Geometry: final body of the model. Coordinates: model frame, mm. A direction names the side the tool comes from. Give positions to 0.01 mm unless a question says otherwise; leave off trailing zeros. Loops run counter-clockwise (first coordinate to the right, second up) from the corner with the lowest first, then second, coordinate; pieces in that order, holes last.
1. Section A-A, the plane x = 135. Output: boundary loops of the cut face in (y, z), then the cut area to 3 significant figures.
2. Material intervals for line 1 along X through (y, z) = (3.25, -9); line 2 along Y through (x, z) = (135, -76.8); line 3 along X through (y, z) = (5, -88.25), sorted ascending.
3. Access query for faces 5 (the face through (15, 5, -15)), 6 (the face through (74, 10, -46)), 7 (the face through (131, 5, -82)), 8 (the face through (74, 5, -90)), 9 (the face through (137.86, 4.1, -77.41)). Directions: +Z, -Z, +X, -X, +Y, -Y. A direction counts if a zero-diameter tool reaches every point of the face in a straight line with its end or side. Return the directions, or none.
4. First-contact query: P1, Ø3, axis at x = 15, y = 5, coming from the -Z side; P2, Ø3.5, axis at x = 135, y = 5, coming from the +Z side. Flat tips, straight axial feed; report the tip coordinate or a pass-through.
5. Draft query along Z for faces 1 (the face through (74, 5, 0)), 2 (the face through (131, 5, -8)), 3 (the face through (135, 5, -75)), 4 (the face through (0, 5, -44)). Return one class per face: +Z half, -Z half, draft (parallel to the pull), parting line (faces both ways), or undercut.
from build123d import *

# Parameters (mm, degrees)
SKETCH1_W           = 150
SKETCH1_H           = 90
SKETCH1_W_2         = 8
SKETCH1_H_2         = 4
BOSS_EXTRUDE1_DEPTH = 10
SKETCH3_R           = 3
CUT_EXTRUDE1_DEPTH  = 15
CUT_EXTRUDE2_START  = -15
SKETCH4_R           = 3
CUT_EXTRUDE2_DEPTH  = 15


with BuildPart() as part:
    # Sketch1 → Boss-Extrude1 (new body)
    with BuildSketch(Plane(origin=(0, 0, 0), x_dir=(1, 0, 0), z_dir=(0, 1, 0))):
        with Locations((75, 45)):
            Rectangle(SKETCH1_W, SKETCH1_H)
        with Locations((135, 8.120559305)):
            Rectangle(SKETCH1_W_2, SKETCH1_H_2, mode=Mode.SUBTRACT)
        with Locations((15, 81.879440695)):
            Rectangle(SKETCH1_W_2, SKETCH1_H_2, mode=Mode.SUBTRACT)
        with Locations((135, 81.879440695)):
            Rectangle(SKETCH1_W_2, SKETCH1_H_2, mode=Mode.SUBTRACT)
        with Locations((15, 8.120559305)):
            Rectangle(SKETCH1_W_2, SKETCH1_H_2, mode=Mode.SUBTRACT)
    extrude(amount=BOSS_EXTRUDE1_DEPTH)

    # Sketch3 → Cut-Extrude1 (cut)
    with BuildSketch(Plane.XY):
        with Locations((15, 5)):
            Circle(SKETCH3_R)
        with Locations((135, 5)):
            Circle(SKETCH3_R)
    extrude(amount=-CUT_EXTRUDE1_DEPTH, mode=Mode.SUBTRACT)

    # Sketch4 → Cut-Extrude2 (cut)
    with BuildSketch(Plane(origin=(0, 0, -90), x_dir=(-1, 0, 0), z_dir=(0, 0, -1)).offset(CUT_EXTRUDE2_START)):
        with Locations(Location((-15, 5, 0), (0, 0, 180))):
            Circle(SKETCH4_R)
        with Locations(Location((-135, 5, 0), (0, 0, 180))):
            Circle(SKETCH4_R)
    extrude(amount=CUT_EXTRUDE2_DEPTH, mode=Mode.SUBTRACT)


solid = part.part
Answers below:
1. outline: (0, -90) - (2, -90) - (2, -83.88) - (0, -83.88) - close; (0, -79.88) - (2, -79.88) - (2, -75) - (8, -75) - (8, -79.88) - (10, -79.88) - (10, -10.12) - (8, -10.12) - (8, -15) - (2, -15) - (2, -10.12) - (0, -10.12) - close; (0, -6.12) - (2, -6.12) - (2, 0) - (0, 0) - close; (8, -90) - (10, -90) - (10, -83.88) - (8, -83.88) - close; (8, -6.12) - (10, -6.12) - (10, 0) - (8, 0) - close
1. area: 688 mm2
2. line 1: x = 0 to 11, 19 to 131, 139 to 150
2. line 2: y = 0 to 2, 8 to 10
2. line 3: x = 0 to 12, 18 to 132, 138 to 150
3. face 5: +Z
3. face 6: +Z, -Z, +X, -X, +Y
3. face 7: +Y, -Y
3. face 8: -Z, +X, -X, +Y, -Y
3. face 9: -Z
4. P1: stops at z = -75
4. P2: stops at z = -15
5. face 1: +Z half
5. face 2: undercut
5. face 3: -Z half
5. face 4: draft
